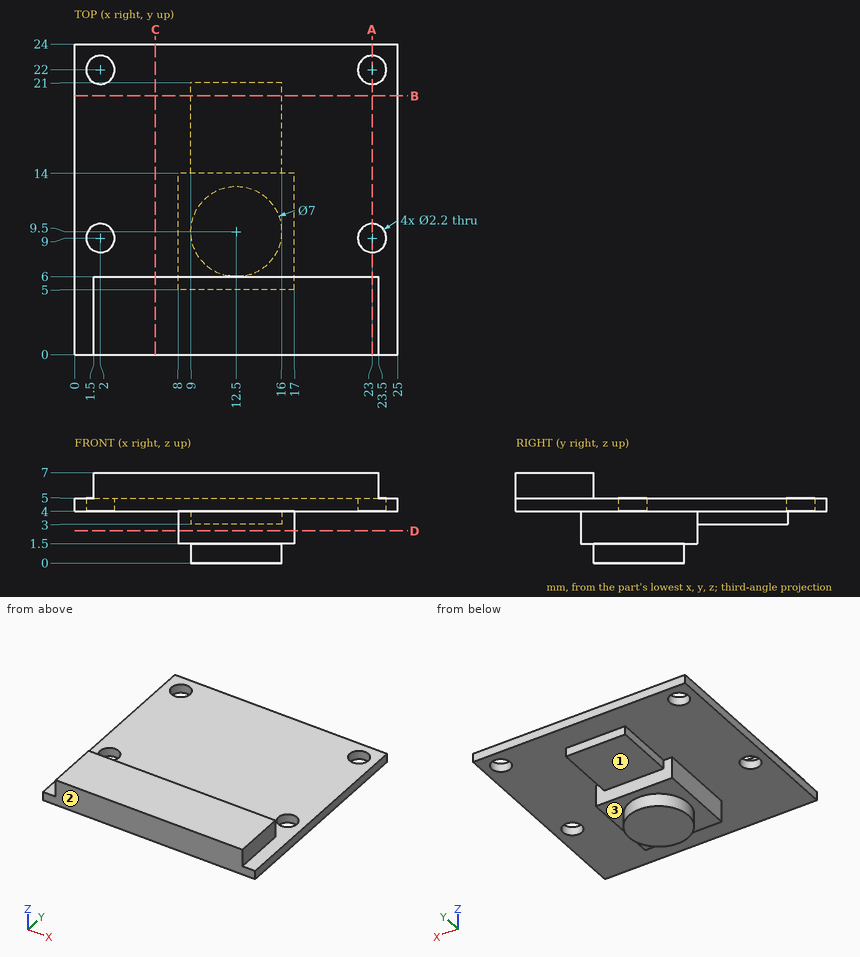
Here's the drawing with two shaded views (mm, measured from the low corner). I have some questions. A direction names the side the tool comes from. Coordinates: 2 decimals unless noted, no trailing zeros. Write each loop counter-clockwise with the first axis right and the second up, starting at its lowest first coordinate (ties: lowest second). Pieces come first, ordered by that corner, then holes.
Item 1: I want a section at C-C on x = 6.25. Write out the boundary of the cut face in (y, z), and give its area (3 significant figures).
Item 2: If I drill on line 1 (Y direction, x = 23, z = 4.55); line 2 (Z direction, x = 4.75, y = 11.25); line 3 (Y direction, x = 11, z = 3.5), over which ranges is the centre line in solid material (lowest first)?
Item 3: I want a section at A-A on x = 23. Write out the boundary of the cut face in (y, z).
Item 4: I want a section at B-B on y = 20. Write out the boundary of the cut face in (x, z), and give its area (3 significant figures).
Item 5: Will these pins go through, and if not, where does the flat tip stop? pin 1 (1.5 mm diameter, centred on x = 22, y = 8.5, fed in from +Z); pin 2 (0.5 mm diameter, centred on x = 13, z = 3.5, fed in from +Y); pin 3 (1 mm diameter, centred on x = 3, y = 18.5, fed in from -Z).
Item 6: On a 3-axis mill with a long thin cutter (end or side, diameter ignored), from which of +Z, -Z, +X, -X, +Y, -Y can I reach the whole of each face in a straight line? I mean the marked faces 1, 2 and 3. Say none if no direction works.
Item 7: I want a section at D-D on z = 2.5. Write out the boundary of the cut face in (x, y).
Findings below:
1. outline: (0, 4) - (24, 4) - (24, 5) - (6, 5) - (6, 7) - (0, 7) - close
1. area: 36.0 mm2
2. line 1: y = 0 to 7.9, 10.1 to 20.9, 23.1 to 24
2. line 2: z = 4 to 5
2. line 3: y = 5 to 21
3. outline: (0, 4) - (7.9, 4) - (7.9, 5) - (6, 5) - (6, 7) - (0, 7) - close; (10.1, 4) - (20.9, 4) - (20.9, 5) - (10.1, 5) - close; (23.1, 4) - (24, 4) - (24, 5) - (23.1, 5) - close
4. outline: (0, 4) - (9, 4) - (9, 3) - (16, 3) - (16, 4) - (25, 4) - (25, 5) - (0, 5) - close
4. area: 32.0 mm2
5. pin 1: stops at z = 5
5. pin 2: stops at y = 21
5. pin 3: stops at z = 4
6. face 1: -Z, +X, -X, +Y
6. face 2: +Z, -Z, +X, -X, -Y
6. face 3: -Z
7. outline: (8, 5) - (17, 5) - (17, 14) - (8, 14) - close
